from build123d import *

# Parameters (mm, degrees)
BOSS_EXTRUDE1_DEPTH     = 20
SKETCH2_W               = 19.610643165
SKETCH2_H               = 11
CUT_EXTRUDE1_DEPTH      = 227.167829004
CUT_EXTRUDE1_DEPTH_BACK = 227.167829004
SKETCH7_R               = 11
CUT_EXTRUDE2_DEPTH      = 10.5
SKETCH6_W               = 2.5
SKETCH6_H               = 6.937111225


with BuildPart() as part:
    # Sketch1 → Boss-Extrude1 (new body)
    with BuildSketch(Plane(origin=(0, 0, 0), x_dir=(1, 0, 0), z_dir=(0, 1, 0))):
        with BuildLine():
            Line((-14.599777392, -163.687024017), (-14.599777392, -179.289222575))
            ThreePointArc((-14.599777392, -179.289222575), (-13.212758245, -184.889636615), (-9.372337822, -189.195403737))
            Line((-9.372337822, -189.195403737), (-4.197358995, -192.733382325))
            ThreePointArc((-4.197358995, -192.733382325), (0.923201568, -198.474405155), (2.772560431, -205.941623874))
            Line((2.772560431, -205.941623874), (2.772560431, -208.068159927))
            ThreePointArc((2.772560431, -208.068159927), (4.572718915, -222.13666845), (-8, -215.572352665))
            Line((-8, -215.572352665), (-8, -208.969123671))
            ThreePointArc((-8, -208.969123671), (-9.205712947, -200.564063539), (-17, -197.195403737))
            ThreePointArc((-17, -197.195403737), (-22.656854249, -194.852257987), (-25, -189.195403737))
            Line((-25, -189.195403737), (-25, -177.754249464))
            Line((-25, -177.754249464), (-27.7, -177.754249464))
            Line((-27.7, -177.754249464), (-27.7, -174.754249464))
            Line((-27.7, -174.754249464), (-25, -174.754249464))
            Line((-25, -174.754249464), (-25, -171.754249464))
            Line((-25, -171.754249464), (-27.7, -171.754249464))
            Line((-27.7, -171.754249464), (-27.7, -168.754249464))
            Line((-27.7, -168.754249464), (-25, -168.754249464))
            Line((-25, -168.754249464), (-25, -165.754249464))
            Line((-25, -165.754249464), (-27.7, -165.754249464))
            Line((-27.7, -165.754249464), (-27.7, -162.754249464))
            Line((-27.7, -162.754249464), (-25, -162.754249464))
            Line((-25, -162.754249464), (-25, -159.754249464))
            Line((-25, -159.754249464), (-27.7, -159.754249464))
            Line((-27.7, -159.754249464), (-27.7, -156.754249464))
            Line((-27.7, -156.754249464), (-25, -156.754249464))
            Line((-25, -156.754249464), (-25, -153.754249464))
            Line((-25, -153.754249464), (-27.7, -153.754249464))
            Line((-27.7, -153.754249464), (-27.7, -150.754249464))
            Line((-27.7, -150.754249464), (-25, -150.754249464))
            Line((-25, -150.754249464), (-20.599777392, -153.294719172))
            ThreePointArc((-20.599777392, -153.294719172), (-16.207472546, -157.687024017), (-14.599777392, -163.687024017))
        make_face()
    extrude(amount=BOSS_EXTRUDE1_DEPTH)

    # Sketch2 → Cut-Extrude1 (cut, two sides)
    with BuildSketch(Plane(origin=(0, 0, 0), x_dir=(0, 0, -1), z_dir=(1, 0, 0))) as cut_extrude1_sk:
        with Locations((-215.877674248, 5)):
            Rectangle(SKETCH2_W, SKETCH2_H)
    extrude(amount=CUT_EXTRUDE1_DEPTH, mode=Mode.SUBTRACT)
    extrude(cut_extrude1_sk.sketch, amount=-CUT_EXTRUDE1_DEPTH_BACK, mode=Mode.SUBTRACT)

    # Sketch4 → Cut-Revolve8 (revolve, cut)
    with BuildSketch(Plane(origin=(0, 0, 0), x_dir=(0, 0, -1), z_dir=(1, 0, 0)), mode=Mode.PRIVATE) as cut_revolve8_sk:
        Polygon((-213.371823115, 3.99935592), (-216.352696282, 4.00886504), (-216.352696282, 9.999898237), (-216.352696282, 21.744358227), (-211.315205583, 21.744358227), (-211.327201493, 17.983937872), (-213.333571374, 15.990328105), (-213.352711547, 9.990358634), align=None)
    revolve(cut_revolve8_sk.sketch.rotate(Axis((0, 4.00886504, 216.352696282), (0, 1, 0)), 180), axis=Axis((0, 4.00886504, 216.352696282), (0, 1, 0)), mode=Mode.SUBTRACT)

    # Sketch7 → Cut-Extrude2 (cut)
    with BuildSketch(Plane(origin=(0, 20, 0), x_dir=(1, 0, 0), z_dir=(0, 1, 0))):
        with Locations((-17, -189.195403737)):
            Circle(SKETCH7_R)
    extrude(amount=-CUT_EXTRUDE2_DEPTH, mode=Mode.SUBTRACT)

    # Sketch6 → Revolve2 (revolve)
    with BuildSketch(Plane.XY.offset(189.195403737)):
        Polygon((-17, 10), (-14.5, 10), (-14.5, 16.207106781), (-12.5, 18.207106781), (-12.5, 20), (-17, 20), align=None)
        with Locations((-15.75, 6.531444388)):
            Rectangle(SKETCH6_W, SKETCH6_H)
        Polygon((-14, 16), (-14, 10), (-9, 10), (-9, 20), (-12, 20), (-12, 18), align=None)
    revolve(axis=Axis((-17, 0, 189.195403737), (0, 1, 0)))


with BuildPart() as revolve2_kept_piece:
    # of the separate pieces the step leaves, the one the design keeps (revolve2_pieces_kept)
    add(part.part.solids().sort_by_distance((-25, 0, 189.195403737))[0])


solid = revolve2_kept_piece.part
The listing builds one solid part. Answer for the finished solid, in the listing's coordinates (mm). A direction names the side the tool comes from. Round coordinates to 2 decimals unless told otherwise and drop trailing zeros. Put each result on its own line as item: value.
Q1. Section A-A, the plane y = 14 is taken. Count the separate pieces of the cut face and the enclosed holes in it, and give its area (3 significant figures).
Results list:
separate pieces: 3
enclosed holes: 1
area: 641 mm^2
Q2. Determine the mould class of faces 4 (the flat face through (-20, 9.5, 188)), 5 (the flat face through (0, 10.5, 213)), 6 (the cylindrical face through (0.872, 9.86, 198.378)) for opening direction Y: pulls with the +Y half, pulls with the -Y half, needs draft (parallel to the pull), parting line crosses it, or undercut.
Results list:
face 4: undercut
face 5: pulls with the -Y half
face 6: needs draft
Q3. Which of the six approach directions +Z, -Z, +X, -X, +Y, -Y give full straight-line access (tool end or side, diameter ignored) to faces 1 (the flat face through (-25, 10, 173)), 2 (the conical face through (-15.79, 16.33, 191.52)), 3 (the flat face through (-14.6, 10, 171))?
Results list:
face 1: -X, +Y, -Y
face 2: none
face 3: -Z, +X, +Y, -Y
Q4. Each of these flat-tipped pins is pushed along its axis until it touches: P1, Ø0.8, axis at x = -26.5, y = 10.5, coming from the +Z side; P2, Ø3.5, axis at y = 8.5, z = 183.5, coming from the -X side; P3, Ø2, axis at x = 1.5, y = 15, coming from the +Z side. Where does it stop, or does it pass through?
Results list:
P1: z = 177.75
P2: x = -25
P3: z = 223.56
Q5. Consider line 1 along Y through (x, z) = (-5, 213.5); line 2 along Z through (x, y) = (-19, 17.25); line 3 along X through (y, z) = (7.25, 172). Determine where each line is inside the solid, lowest interval first.
Results list:
line 1: 10.5 to 20
line 2: 154.4 to 178.38, 186.27 to 192.12
line 3: -25 to -14.6
